Can you work these out from the model? Positions are in its coordinate system, mm. A direction names the side the tool comes from. Coordinates: 2 decimals unless noted, no trailing zeros. Loops run counter-clockwise (first coordinate to the right, second up) from the corner with the lowest first, then second, coordinate; pieces in that order, holes last.
```python
from build123d import *

# Parameters (mm, degrees)
SKETCH1_W               = 45
SKETCH1_H               = 30
SKETCH1_R               = 2.15
SKETCH1_R_2             = 5
BOSS_EXTRUDE1_DEPTH     = 3
SKETCH3_W               = 20
SKETCH3_H               = 5
EXTRUDE_THIN1_DEPTH     = 10
CUT_EXTRUDE1_DEPTH      = 41.746165464
BOSS_EXTRUDE2_DEPTH     = 2
SKETCH6_W               = 3
SKETCH6_H               = 15
CUT_EXTRUDE2_DEPTH      = 48.013295992
CHAMFER2_SIZE           = 6
CHAMFER1_SIZE           = 10
SKETCH8_R               = 4.5
SKETCH8_R_2             = 2.5
EXTRUDE_THIN3_DEPTH     = 2.5
MOVE_START              = -27.5
MOVE_FACE1_DEPTH        = 7.5
MOVE_FACE1_2_DEPTH      = 2.5
CUT_EXTRUDE3_DEPTH      = 43.32611487
CUT_EXTRUDE3_DEPTH_BACK = 43.32611487
SKETCH11_R              = 7.5
FILLET1_R               = 3


# Read off the part's stored shape, not the designer's step: Move Face1
with BuildPart() as part:
    # Sketch1 → Boss-Extrude1 (new body)
    with BuildSketch(Plane.XY):
        with Locations((0, -10)):
            Rectangle(SKETCH1_W, SKETCH1_H)
        with Locations((-17.5, 0)):
            Circle(SKETCH1_R, mode=Mode.SUBTRACT)
        with Locations(Location((17.5, 0, 0), (0, 0, 180))):
            Circle(SKETCH1_R, mode=Mode.SUBTRACT)
        with Locations((0, -8)):
            Circle(SKETCH1_R_2, mode=Mode.SUBTRACT)
    extrude(amount=BOSS_EXTRUDE1_DEPTH)

    # Sketch3 → Extrude-Thin1 (add, symmetric)
    with BuildSketch(Plane.ZY):
        with Locations((13, -22.5)):
            Rectangle(SKETCH3_W, SKETCH3_H)
    extrude(amount=EXTRUDE_THIN1_DEPTH, both=True)

    # Sketch4 → Cut-Extrude1 (cut, through all)
    with BuildSketch(Plane(origin=(0, -20, 0), x_dir=(1, 0, 0), z_dir=(0, 1, 0))):
        with BuildLine():
            Line((-2, -14.5), (2, -14.5))
            ThreePointArc((2, -14.5), (2.5, -16), (2, -17.5))
            Line((2, -17.5), (-2, -17.5))
            ThreePointArc((-2, -17.5), (-2.5, -16), (-2, -14.5))
        make_face()
    extrude(amount=-CUT_EXTRUDE1_DEPTH, mode=Mode.SUBTRACT)

    # Sketch5 → Boss-Extrude2 (add)
    with BuildSketch(Plane.ZY.offset(10)):
        Polygon((23, -20), (3, 0), (3, -20), align=None)
    boss_extrude2 = extrude(amount=-BOSS_EXTRUDE2_DEPTH)

    # Sketch6 → Cut-Extrude2 (cut, through all)
    with BuildSketch(Plane.ZY.offset(10)):
        with Locations((1.5, -17.5)):
            Rectangle(SKETCH6_W, SKETCH6_H)
    cut_extrude2 = extrude(amount=CUT_EXTRUDE2_DEPTH, mode=Mode.SUBTRACT)

    # Mirror1: Boss-Extrude2, Cut-Extrude2 across plane
    add(boss_extrude2.mirror(Plane(origin=(0, 0, 0), x_dir=(0, 0, 1), z_dir=(1, 0, 0))))
    add(cut_extrude2.mirror(Plane(origin=(0, 0, 0), x_dir=(0, 0, 1), z_dir=(1, 0, 0))), mode=Mode.SUBTRACT)

    # Chamfer2
    chamfer2_edges = [part.edges().sort_by_distance(p)[0] for p in [
        (0, -20, 3),
    ]]
    chamfer(chamfer2_edges, length=CHAMFER2_SIZE)

    # Chamfer1
    chamfer1_edges = [part.edges().sort_by_distance(p)[0] for p in [
        (0, -25, 0),
    ]]
    chamfer(chamfer1_edges, length=CHAMFER1_SIZE)

    # Sketch8 → Extrude-Thin3 (add)
    with BuildSketch(Plane.XZ.offset(25)):
        with Locations((0, 16)):
            Circle(SKETCH8_R)
        with Locations((0, 16)):
            Circle(SKETCH8_R_2, mode=Mode.SUBTRACT)
    extrude(amount=EXTRUDE_THIN3_DEPTH)

    # Move Face1 outline → Move Face1 (cut)
    with BuildSketch(Plane(origin=(0, 0, 0), x_dir=(1, 0, 0), z_dir=(0, 1, 0)).offset(MOVE_START)):
        with BuildLine():
            ThreePointArc((2.049390153, -17.6), (2.6, -16), (2.049390153, -14.4))
            Line((2.049390153, -14.4), (-2.049390153, -14.4))
            ThreePointArc((-2.049390153, -14.4), (-2.6, -16), (-2.049390153, -17.6))
            Line((-2.049390153, -17.6), (2.049390153, -17.6))
        make_face()
        with BuildLine():
            Line((2, -17.5), (-2, -17.5))
            ThreePointArc((-2, -17.5), (-2.5, -16), (-2, -14.5))
            Line((-2, -14.5), (2, -14.5))
            ThreePointArc((2, -14.5), (2.5, -16), (2, -17.5))
        make_face(mode=Mode.SUBTRACT)
    extrude(amount=MOVE_FACE1_DEPTH, mode=Mode.SUBTRACT)

    # Move Face1 2 outline → Move Face1 2 (cut)
    with BuildSketch(Plane(origin=(0, 0, 0), x_dir=(1, 0, 0), z_dir=(0, 1, 0)).offset(MOVE_START)):
        with BuildLine():
            Line((1.920937271, -14.4), (2.049390153, -14.4))
            ThreePointArc((2.049390153, -14.4), (0, -13.4), (-2.049390153, -14.4))
            Line((-2.049390153, -14.4), (-1.920937271, -14.4))
            ThreePointArc((-1.920937271, -14.4), (0, -13.5), (1.920937271, -14.4))
        make_face()
        with BuildLine():
            ThreePointArc((-2.049390153, -17.6), (0, -18.6), (2.049390153, -17.6))
            Line((2.049390153, -17.6), (1.920937271, -17.6))
            ThreePointArc((1.920937271, -17.6), (0, -18.5), (-1.920937271, -17.6))
            Line((-1.920937271, -17.6), (-2.049390153, -17.6))
        make_face()
    extrude(amount=MOVE_FACE1_2_DEPTH, mode=Mode.SUBTRACT)

    # Sketch11 → Cut-Extrude3 (cut, two sides: drawn at the far end of the back side and taken through both)
    with BuildSketch(Plane(origin=(0, 0, 0), x_dir=(0, 0, -1), z_dir=(1, 0, 0)).offset(-CUT_EXTRUDE3_DEPTH_BACK)):
        with Locations((-16, -8)):
            Circle(SKETCH11_R)
    extrude(amount=CUT_EXTRUDE3_DEPTH + CUT_EXTRUDE3_DEPTH_BACK, mode=Mode.SUBTRACT)

    # Fillet1
    fillet1_edges = [part.edges().sort_by_distance(p)[0] for p in [
        (0, -20, 9),
        (0, -14, 3),
        (0, -25, 10),
        (0, -15, 0),
        (-9, -15.177071733, 18.177071733),
        (-9, -5.822928267, 8.822928267),
        (9, -15.177071733, 18.177071733),
        (9, -5.822928267, 8.822928267),
        (-10, -10, 1.5),
        (-22.5, -10, 1.5),
        (-22.5, 5, 1.5),
        (22.5, 5, 1.5),
        (22.5, -10, 1.5),
        (10, -10, 1.5),
    ]]
    fillet(fillet1_edges, radius=FILLET1_R)


solid = part.part
```
Item 1: I need wall thicknesses on line 1 along Y through (x, z) = (17.5, 1.5); line 2 along X through (y, z) = (-6.5, 6.25); line 3 along Z through (x, y) = (4, 1). Which ranges of each line are inside material? Lowest first, please.
Results are:
line 1: y = -10 to -2.15, 2.15 to 5
line 2: x = -10 to -8, 8 to 10
line 3: z = 0 to 3
Item 2: Suppose I cut it at C-C, the plane z = 21.25. Please give me the cut outline in (x, y).
Results are:
outline: (-10, -25) - (10, -25) - (10, -18.25) - (8, -18.25) - (8, -20) - (-8, -20) - (-8, -18.25) - (-10, -18.25) - close
Item 3: On a 3-axis mill with a long thin cutter (end or side, diameter ignored), from which of +Z, -Z, +X, -X, +Y, -Y can I reach the whole of each face in a straight line? I mean faces 4 (the face through (-4.72, -13.89, 3.22)), 5 (the face through (-0.59, -26.23, 20.46)), 6 (the face through (-16, -10, 1)), 7 (the face through (16, -10, 1)). Say none if no direction works.
Results are:
face 4: +Z, +Y
face 5: -Y
face 6: +Z, -Z, -X, -Y
face 7: +Z, -Z, +X, -Y
Item 4: Suppose I cut it at B-B, the plane x = 17.5. Please give me the cut outline in (y, z), plus the area to 3 significant figures.
Results are:
outline: (-10, 0) - (-2.15, 0) - (-2.15, 3) - (-10, 3) - close; (2.15, 0) - (5, 0) - (5, 3) - (2.15, 3) - close
area: 32.1 mm2
Item 5: Suppose I cut it at D-D, the plane y = -1. Please give me the cut outline in (x, z).
Results are:
outline: (-22.5, 0) - (-19.4, 0) - (-19.4, 3) - (-22.5, 3) - close; (-15.6, 0) - (15.6, 0) - (15.6, 3) - (10, 3) - (10, 4) - (8, 4) - (8, 3) - (-8, 3) - (-8, 4) - (-10, 4) - (-10, 3) - (-15.6, 3) - close; (19.4, 0) - (22.5, 0) - (22.5, 3) - (19.4, 3) - close
Item 6: Suppose I cut it at A-A, the plane y = -8. Please give me the cut outline in (x, z).
Results are:
outline: (-22.33, 0) - (-5, 0) - (-5, 3) - (-8, 3) - (-8, 8.5) - (-10, 8.5) - (-10, 3) - (-22.33, 3) - close; (5, 0) - (22.33, 0) - (22.33, 3) - (10, 3) - (10, 8.5) - (8, 8.5) - (8, 3) - (5, 3) - close
Item 7: I'm going to push flat-ended pins straight in: P1, Ø0.5, axis at x = -0.5, z = 18, coming from the -Y side; P2, Ø2, axis at x = 4, z = 13, coming from the +Y side; P3, Ø1, axis at x = -5, z = 5, coming from the +Y side; P4, Ø10, axis at y = -8.5, z = 17.5, coming from the +X side. Where does each tip first touch, or does it pass through?
Results are:
P1: stops at y = -25
P2: stops at y = -20
P3: stops at y = -15.5
P4: passes through
Item 8: We'd pull the mould along Z, two halves only. Please class faces 1 (the face through (0, -25, 21)), 2 (the face through (0, -20, 5)), 3 (the face through (0, -23, 17.6)): +Z half, -Z half, draft (parallel to the pull), parting line (faces both ways), or undercut.
Results are:
face 1: draft
face 2: -Z half
face 3: undercut
